```python
from build123d import *

# Parameters (mm, degrees)
SKETCH1_W           = 13.3
SKETCH1_H           = 11.35
BOSS_EXTRUDE1_DEPTH = 9.7
SKETCH2_R           = 3.6
BOSS_EXTRUDE2_DEPTH = 7
SKETCH3_R           = 3
BOSS_EXTRUDE4_DEPTH = 13
SKETCH4_W           = 2
SKETCH4_H           = 0.8
BOSS_EXTRUDE5_DEPTH = 0.8


with BuildPart() as part:
    # Sketch1 → Boss-Extrude1 (new body)
    with BuildSketch(Plane.XY):
        with Locations((6.65, 5.675)):
            Rectangle(SKETCH1_W, SKETCH1_H)
    extrude(amount=BOSS_EXTRUDE1_DEPTH)

    # Sketch2 → Boss-Extrude2 (add)
    with BuildSketch(Plane(origin=(13.3, 0, 0), x_dir=(0, 0, -1), z_dir=(1, 0, 0))):
        with Locations(Location((-4.85, 6.5, 0), (0, 0, 270))):  # turned: the seam where the file's is
            Circle(SKETCH2_R)
    extrude(amount=BOSS_EXTRUDE2_DEPTH)

    # Sketch3 → Boss-Extrude4 (add)
    with BuildSketch(Plane(origin=(20.3, 0, 0), x_dir=(0, 0, -1), z_dir=(1, 0, 0))):
        with Locations(Location((-4.85, 6.5, 0), (0, 0, 270))):  # turned: the seam where the file's is
            Circle(SKETCH3_R)
    extrude(amount=BOSS_EXTRUDE4_DEPTH)

    # Sketch4 → Boss-Extrude5 (add)
    with BuildSketch(Plane(origin=(13.3, 0, 0), x_dir=(0, 0, -1), z_dir=(1, 0, 0))):
        with Locations((-4.85, 0.4)):
            Rectangle(SKETCH4_W, SKETCH4_H)
    extrude(amount=BOSS_EXTRUDE5_DEPTH)


solid = part.part
```
Source: CAD feature listing. Evaluate the final solid. Frame: model axes, mm. A direction names the side the tool comes from. Give positions to 0.01 mm unless a question says otherwise; leave off trailing zeros. Order: outer loops, then holes, each group sorted by start corner. A loop starts at its lowest first (then second) coordinate and runs counter-clockwise, first axis right, second up. Notation, with made-up numbers: (73, 48.5) -> (115, 48.5) arc R19 ccw to (115, 80.5) -> close; hole circle Ø5 at (-15.75, 36.5). An arc over 180 degrees is marked (long way). Use a Markdown table: item, result.
Q1. Section C-C (x = 22). Return the cut outline in (y, z).
A:
| item | result |
|---|---|
| outline | circle Ø6 at (6.5, 4.85) |
Q2. Material intervals for line 1 (X direction, y = 1, z = 6.75); line 2 (X direction, y = 7, z = 8); line 3 (Y direction, x = 28.5, z = 2.5), sorted ascending. Write a range as [from, to].
A:
| item | result |
|---|---|
| line 1 | [0, 13.3] |
| line 2 | [0, 20.3] |
| line 3 | [4.64, 8.36] |
Q3. Pull-direction query (Y, two-part tool) for faces 3 (the face through (7, 6, 9.7)), 4 (the face through (13.7, 0.8, 4.9)), 5 (the face through (7, 0, 5)); classes: +Y half, -Y half, draft (parallel to the pull), parting line (faces both ways), or undercut.
A:
| item | result |
|---|---|
| face 3 | draft |
| face 4 | undercut |
| face 5 | -Y half |
Q4. Section A-A (z = 4.85). Return the cut outline in (x, y).
A:
| item | result |
|---|---|
| outline | (0, 0) -> (14.1, 0) -> (14.1, 0.8) -> (13.3, 0.8) -> (13.3, 2.9) -> (20.3, 2.9) -> (20.3, 3.5) -> (33.3, 3.5) -> (33.3, 9.5) -> (20.3, 9.5) -> (20.3, 10.1) -> (13.3, 10.1) -> (13.3, 11.35) -> (0, 11.35) -> close |
Q5. Access query for faces 1 (the face through (33.3, 7, 5)), 2 (the face through (17, 3, 4)). Directions: +Z, -Z, +X, -X, +Y, -Y. A direction counts if a zero-diameter tool reaches every point of the face in a straight line with its end or side. Return the directions, or none.
A:
| item | result |
|---|---|
| face 1 | +Z, -Z, +X, +Y, -Y |
| face 2 | +X |
Q6. Section D-D (z = 7.5). Return the cut outline in (x, y).
A:
| item | result |
|---|---|
| outline | (0, 0) -> (13.3, 0) -> (13.3, 4.06) -> (20.3, 4.06) -> (20.3, 5.09) -> (33.3, 5.09) -> (33.3, 7.91) -> (20.3, 7.91) -> (20.3, 8.94) -> (13.3, 8.94) -> (13.3, 11.35) -> (0, 11.35) -> close |
Q7. Section B-B (y = 6.5). Return the cut outline in (x, z).
A:
| item | result |
|---|---|
| outline | (0, 0) -> (13.3, 0) -> (13.3, 1.25) -> (20.3, 1.25) -> (20.3, 1.85) -> (33.3, 1.85) -> (33.3, 7.85) -> (20.3, 7.85) -> (20.3, 8.45) -> (13.3, 8.45) -> (13.3, 9.7) -> (0, 9.7) -> close |
Q8. First-contact query: P1, Ø2, axis at x = 18, y = 5, coming from the -Z side; P2, Ø0.6, axis at y = 0, z = 4.5, coming from the +X side. Flat tips, straight axial feed; report the tip coordinate or a pass-through.
A:
| item | result |
|---|---|
| P1 | z = 1.28 |
| P2 | x = 14.1 |
